from build123d import *

# Parameters (mm, degrees)
SKETCH2_W               = 55.88
SKETCH2_H               = 85.09
FIBERGLASS_PCB_DEPTH    = 1.6
SKETCH3_W               = 7.6
SKETCH3_H               = 5.6
USB_MICRO_B_POWER_DEPTH = 2.4
SKETCH4_W               = 5
SKETCH4_H               = 33.2
BOSS_EXTRUDE3_DEPTH     = 2.6
SKETCH5_W               = 11.4
SKETCH5_H               = 15.1
BOSS_EXTRUDE4_DEPTH     = 6.15
SKETCH6_W               = 20.6
SKETCH6_H               = 2.95
BOSS_EXTRUDE5_DEPTH     = 5.6
SKETCH8_R               = 3.25
BOSS_EXTRUDE6_DEPTH     = 8
SKETCH9_W               = 28.4
SKETCH9_H               = 16.8
BOSS_EXTRUDE7_DEPTH     = 3.9
SKETCH10_W              = 24
SKETCH10_H              = 2.1
BOSS_EXTRUDE8_DEPTH     = 18
SKETCH11_R              = 1.45
CUT_EXTRUDE1_DEPTH      = 67.5955601
SKETCH12_R              = 3.175
BOSS_EXTRUDE9_DEPTH     = 6.35
SKETCH13_W              = 55.88
SKETCH13_H              = 93.98
BOSS_EXTRUDE10_DEPTH    = 1.5875
SKETCH14_R              = 1.45
CUT_EXTRUDE2_DEPTH      = 67.797698548


with BuildPart() as part:
    # Sketch2 → Fiberglass PCB (new body)
    with BuildSketch(Plane(origin=(0, 0, 0), x_dir=(1, 0, 0), z_dir=(0, 1, 0))):
        Rectangle(SKETCH2_W, SKETCH2_H)
    extrude(amount=FIBERGLASS_PCB_DEPTH)

    # Sketch3 → USB Micro-B Power (add)
    with BuildSketch(Plane(origin=(0, 1.6, 0), x_dir=(1, 0, 0), z_dir=(0, 1, 0))):
        with Locations((-20.54, 40.245)):
            Rectangle(SKETCH3_W, SKETCH3_H)
    extrude(amount=USB_MICRO_B_POWER_DEPTH)

    # Sketch4 → Boss-Extrude3 (add)
    with BuildSketch(Plane(origin=(0, 1.6, 0), x_dir=(1, 0, 0), z_dir=(0, 1, 0))):
        with Locations((23.94, 24.945)):
            Rectangle(SKETCH4_W, SKETCH4_H)
    extrude(amount=BOSS_EXTRUDE3_DEPTH)

    # Sketch5 → Boss-Extrude4 (add)
    with BuildSketch(Plane(origin=(0, 1.6, 0), x_dir=(1, 0, 0), z_dir=(0, 1, 0))):
        with Locations((-23.44, -2.505)):
            Rectangle(SKETCH5_W, SKETCH5_H)
    extrude(amount=BOSS_EXTRUDE4_DEPTH)

    # Sketch6 → Boss-Extrude5 (add)
    with BuildSketch(Plane(origin=(0, 1.6, 0), x_dir=(1, 0, 0), z_dir=(0, 1, 0))):
        with Locations((0.01, 30.52)):
            Rectangle(SKETCH6_W, SKETCH6_H)
        with Locations((-17.26, -16.78)):
            Rectangle(SKETCH6_W, SKETCH6_H)
    extrude(amount=BOSS_EXTRUDE5_DEPTH)

    # Sketch8 → Boss-Extrude6 (add)
    with BuildSketch(Plane(origin=(0, 1.6, 0), x_dir=(1, 0, 0), z_dir=(0, 1, 0))):
        with Locations(Location((-20.54, 29.295, 0), (0, 0, 90))):
            Circle(SKETCH8_R)
    extrude(amount=BOSS_EXTRUDE6_DEPTH)

    # Sketch9 → Boss-Extrude7 (add)
    with BuildSketch(Plane.XZ):
        with Locations((1.26, -32.945)):
            Rectangle(SKETCH9_W, SKETCH9_H)
    extrude(amount=BOSS_EXTRUDE7_DEPTH)

    # Sketch10 → Boss-Extrude8 (add)
    with BuildSketch(Plane(origin=(0, 0, -41.345), x_dir=(-1, 0, 0), z_dir=(0, 0, -1))):
        with Locations((-1.11, -2.1)):
            Rectangle(SKETCH10_W, SKETCH10_H)
    extrude(amount=BOSS_EXTRUDE8_DEPTH)

    # Sketch11 → Cut-Extrude1 (cut, through all)
    with BuildSketch(Plane(origin=(0, 1.6, 0), x_dir=(1, 0, 0), z_dir=(0, 1, 0))):
        with Locations(Location((15.494, -37.465, 0), (0, 0, 270))):
            Circle(SKETCH11_R)
        with Locations(Location((-9.906, 17.145, 0), (0, 0, 270))):
            Circle(SKETCH11_R)
    extrude(amount=-CUT_EXTRUDE1_DEPTH, mode=Mode.SUBTRACT)

    # Sketch12 → Boss-Extrude9 (add)
    with BuildSketch(Plane.XZ):
        with Locations(Location((-9.906, -17.145, 0), (0, 0, 270))):
            Circle(SKETCH12_R)
        with Locations(Location((15.494, 37.465, 0), (0, 0, 270))):
            Circle(SKETCH12_R)
    extrude(amount=BOSS_EXTRUDE9_DEPTH)

    # Sketch13 → Boss-Extrude10 (add)
    with BuildSketch(Plane.XZ.offset(6.35)):
        with Locations((0, 4.445)):
            Rectangle(SKETCH13_W, SKETCH13_H)
    extrude(amount=BOSS_EXTRUDE10_DEPTH)

    # Sketch14 → Cut-Extrude2 (cut, through all)
    with BuildSketch(Plane(origin=(0, 1.6, 0), x_dir=(1, 0, 0), z_dir=(0, 1, 0))):
        with Locations(Location((-9.906, 17.145, 0), (0, 0, 270))):
            Circle(SKETCH14_R)
        with Locations(Location((15.494, -37.465, 0), (0, 0, 270))):
            Circle(SKETCH14_R)
    extrude(amount=-CUT_EXTRUDE2_DEPTH, mode=Mode.SUBTRACT)


solid = part.part
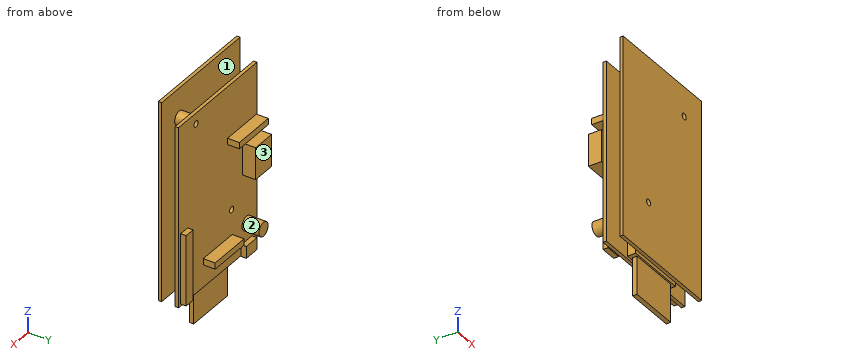
Model file for the job. Use its own axes, mm. Face numbers are marked on the shaded views. Give positions to 0.01 mm unless a question says otherwise; leave off trailing zeros. Order: outer loops, then holes, each group sorted by start corner. A loop starts at its lowest first (then second) coordinate and runs counter-clockwise, first axis right, second up. Notation, with made-up numbers: (-1.75, -24.75) - (33.25, -24.75) arc R18 ccw to (33.25, -20.75) - close; hole circle Ø1 at (43, 81). An arc over 180 degrees is marked (long way). Return JSON: item names as keys, results as strings.
1) Cut at D-D, the plane z = -1. Give the cut face in (x, y).
Geometry says:
{"outline": "(-29.14, 1.6) - (-27.94, 1.6) - (-27.94, 0) - (27.94, 0) - (27.94, 1.6) - (-17.74, 1.6) - (-17.74, 7.75) - (-29.14, 7.75) - close; (-27.94, -7.94) - (27.94, -7.94) - (27.94, -6.35) - (-27.94, -6.35) - close"}
2) Probe line 1 (Y direction, x = -16.5, z = -42.5); line 2 (Z direction, x = -8.5, y = 5) (3 decimals); line 3 (Y direction, x = -17.5, z = -43). List the from-to ranges inside material, lowest first. Write a range as from..to.
Geometry says:
{"line 1": "-7.94..-6.35, 0..1.6", "line 2": "-31.995..-29.045, 15.305..18.255", "line 3": "1.6..4"}
3) Flat gauge pins, fed straight in: P1, Ø2.5, axis at x = -18, z = 17.5, coming from the +Y side; P2, Ø6, axis at x = 0, y = 4, coming from the +Z side (3 decimals); P3, Ø0.8, axis at y = -7, z = -17.5, coming from the -X side. Where does each tip first touch, or does it go through?
Geometry says:
{"P1": "y = 7.2", "P2": "z = 42.545", "P3": "x = -27.94"}
4) Cut at B-B, the plane z = -36. Give the cut face in (x, y).
Geometry says:
{"outline": "(-27.94, -7.94) - (27.94, -7.94) - (27.94, -6.35) - (-27.94, -6.35) - close; (-27.94, 0) - (-12.94, 0) - (-12.94, -3.9) - (15.46, -3.9) - (15.46, 0) - (27.94, 0) - (27.94, 1.6) - (26.44, 1.6) - (26.44, 4.2) - (21.44, 4.2) - (21.44, 1.6) - (-27.94, 1.6) - close"}
5) Pull direction Y, two halves, no side cores. Call the marked faces 1, 2 and 3: pulls with the +Y half, pulls with the -Y half, needs draft (parallel to the pull), parting line crosses it, or undercut.
Geometry says:
{"face 1": "undercut", "face 2": "needs draft", "face 3": "pulls with the +Y half"}
